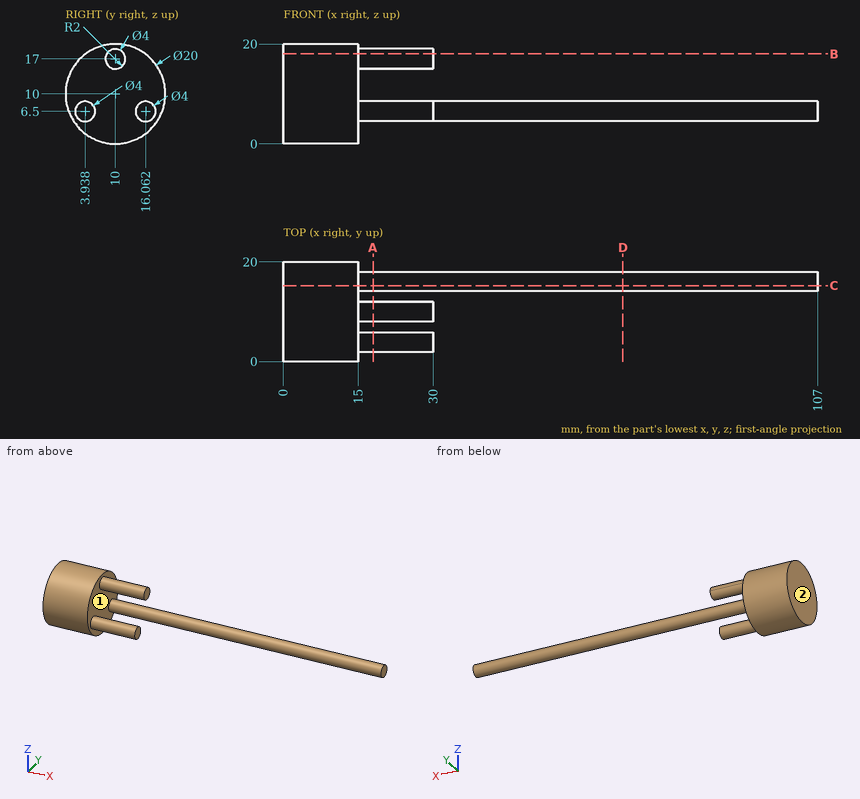
Print and shaded views of the part. All mm, measured from the part's lowest x, y and z. A direction names the side the tool comes from. Coordinates: 2 decimals unless noted, no trailing zeros. Order: outer loops, then holes, each group sorted by start corner. A loop starts at its lowest first (then second) coordinate and runs counter-clockwise, first axis right, second up. Notation, with made-up numbers: M 87,75 L 100,75 A20 cw 100,108 Z; hole C 21.25,70.5 d8. An arc over 180 degrees is marked long. Answer as CSV lines item,"result".
1) 3-axis set-ups, long thin cutter, end or side, ignore diameter. For the marked faces 1 and 2: which of +Z, -Z, +X, -X, +Y, -Y reach the whole face in a straight line?
Verdict:
face 1,"+X"
face 2,"+Z, -Z, -X, +Y, -Y"
2) Flat gauge pins, fed straight in: P1, Ø6, axis at y = 7.5, z = 14, coming from the +X side; P2, Ø5, axis at x = 20.5, y = 15.5, coming from the -Z side; P3, Ø5, axis at x = 73, z = 3.5, coming from the +Y side. Where does each tip first touch, or does it go through?
Verdict:
P1,"x = 30"
P2,"z = 4.5"
P3,"y = 18"
3) Cut at A-A (x = 18). List the corners of the cut face in (y, z).
Verdict:
outline,"C 3.94,6.5 d4; M 10,15 A2 ccw 12,17 A2 ccw long Z; C 16.06,6.5 d4"
4) Cut at B-B (z = 18). List the corners of the cut face in (x, y), then the cut area to 3 significant figures.
Verdict:
outline,"M 0,4 L 15,4 L 15,8.27 L 30,8.27 L 30,11.73 L 15,11.73 L 15,16 L 0,16 Z"
area,"232 mm2"
5) Drill centre lines: L1, parallel to X at y = 3, z = 13; L2, parallel to X at y = 5.25, z = 5.5; L3, parallel to Z at x = 10.5, y = 12. Where is each one in solid material? Low to high. Write a range as from..to.
Verdict:
L1,"0..15"
L2,"0..30"
L3,"0.2..19.8"
6) Cut at D-D (x = 68). List the corners of the cut face in (y, z), then the cut area to 3 significant figures.
Verdict:
outline,"C 16.06,6.5 d4"
area,"12.6 mm2"
7) Cut at C-C (y = 15.25). List the corners of the cut face in (x, z), then the cut area to 3 significant figures.
Verdict:
outline,"M 0,1.49 L 15,1.49 L 15,4.67 L 107,4.67 L 107,8.33 L 15,8.33 L 15,18.51 L 0,18.51 Z"
area,"592 mm2"
